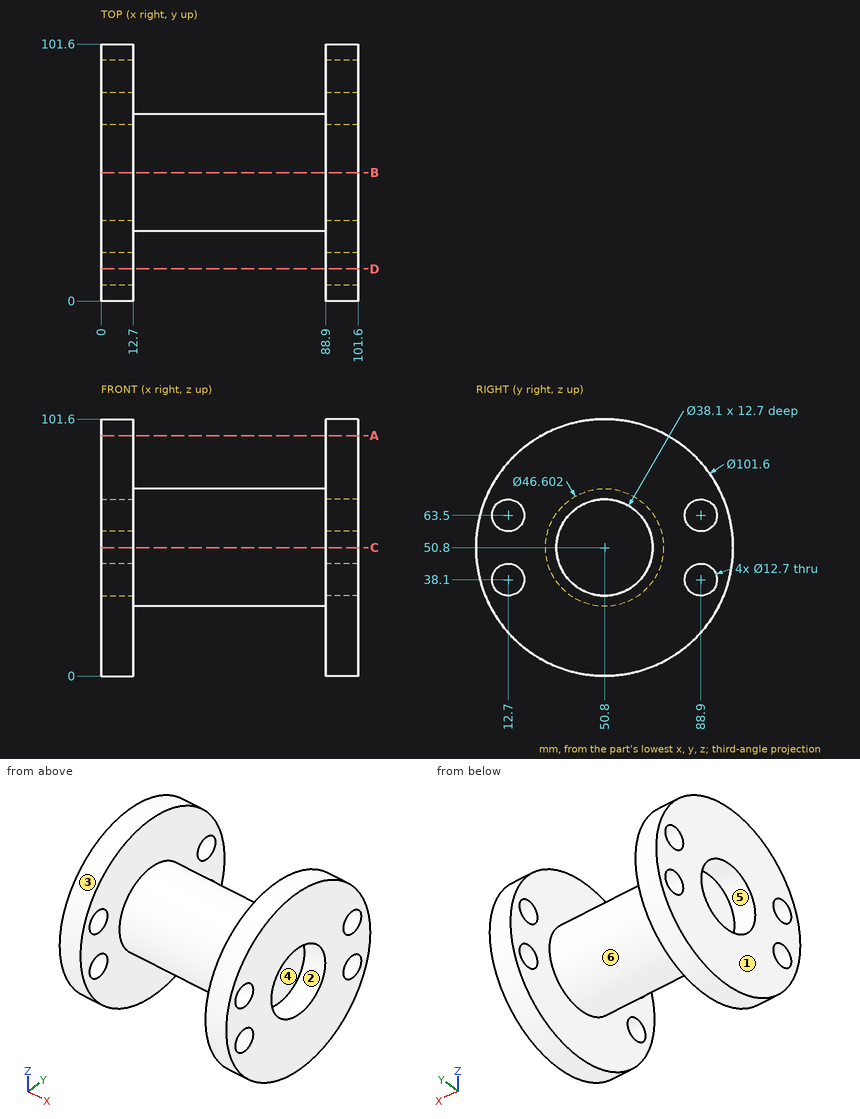
Part print with two shaded views. Sizes in mm from the minimum x, y, z corner. A direction names the side the tool comes from. Round coordinates to 2 decimals unless told otherwise and drop trailing zeros. Order: outer loops, then holes, each group sorted by start corner. A loop starts at its lowest first (then second) coordinate and runs counter-clockwise, first axis right, second up. Notation, with made-up numbers: (33.25, 21) -> (92.25, 21) arc R17 ccw to (92.25, 34) -> close; hole circle Ø5 at (64, 84.25). An arc over 180 degrees is marked (long way). Use one line per item in the form item = value.
Item 1: Drill centre lines: line 1 (X direction, y = 51, z = 12); line 2 (Z direction, x = 92.25, y = 50.8); line 3 (Y direction, x = 10, z = 38). Where is each one in solid material? Low to high.
Returned:
line_1 = 0 to 12.7, 88.9 to 101.6
line_2 = 0 to 31.75, 69.85 to 101.6
line_3 = 1.64 to 6.35, 19.05 to 36.69, 64.91 to 82.55, 95.25 to 99.96
Item 2: Cut at A-A, the plane z = 95. Write the cut outline in (x, y), and give its area (3 significant figures).
Returned:
outline = (0, 25.76) -> (12.7, 25.76) -> (12.7, 75.84) -> (0, 75.84) -> close; (88.9, 25.76) -> (101.6, 25.76) -> (101.6, 75.84) -> (88.9, 75.84) -> close
area = 1,270 mm^2
Item 3: Cut at B-B, the plane y = 50.8. Write the cut outline in (x, z), and give its area (3 significant figures).
Returned:
outline = (0, 0) -> (12.7, 0) -> (12.7, 27.5) -> (88.9, 27.5) -> (88.9, 0) -> (101.6, 0) -> (101.6, 31.75) -> (88.9, 31.75) -> (88.9, 69.85) -> (101.6, 69.85) -> (101.6, 101.6) -> (88.9, 101.6) -> (88.9, 74.1) -> (12.7, 74.1) -> (12.7, 101.6) -> (0, 101.6) -> (0, 69.85) -> (12.7, 69.85) -> (12.7, 31.75) -> (0, 31.75) -> close
area = 5,160 mm^2
Item 4: Tool access for the marked faces 4, 5 and 6: list every direction of +Z, -Z, +X, -X, +Y, -Y with a clear straight run to the whole face (end or side of a thin tool).
Returned:
face_4 = +X
face_5 = -X
face_6 = none
Item 5: Pull direction Z, two halves, no side cores. Call the marked faces 1, 2 and 3: released by +Z, released by -Z, zero draft, split by the parting line, or undercut.
Returned:
face_1 = zero draft
face_2 = undercut
face_3 = split by the parting line
Item 6: Cut at D-D, the plane y = 12.7. Write the cut outline in (x, z).
Returned:
outline = (0, 17.2) -> (12.7, 17.2) -> (12.7, 31.75) -> (0, 31.75) -> close; (0, 44.45) -> (12.7, 44.45) -> (12.7, 57.15) -> (0, 57.15) -> close; (0, 69.85) -> (12.7, 69.85) -> (12.7, 84.4) -> (0, 84.4) -> close; (88.9, 17.2) -> (101.6, 17.2) -> (101.6, 31.75) -> (88.9, 31.75) -> close; (88.9, 44.45) -> (101.6, 44.45) -> (101.6, 57.15) -> (88.9, 57.15) -> close; (88.9, 69.85) -> (101.6, 69.85) -> (101.6, 84.4) -> (88.9, 84.4) -> close
Item 7: Flat gauge pins, fed straight in: pin 1 Ø7.5 at (y, z) = (88.9, 63.5) entering from +X; pin 2 Ø19 at (y, z) = (51.5, 54.5) entering from +X; pin 3 Ø23 at (y, z) = (50.8, 50.8) entering from -X; pin 4 Ø10 at (x, y) = (78.5, 67.5) entering from -Z. Where does each tip first touch, or does it go through?
Returned:
pin_1 = through
pin_2 = 88.9
pin_3 = 12.7
pin_4 = 30.65
